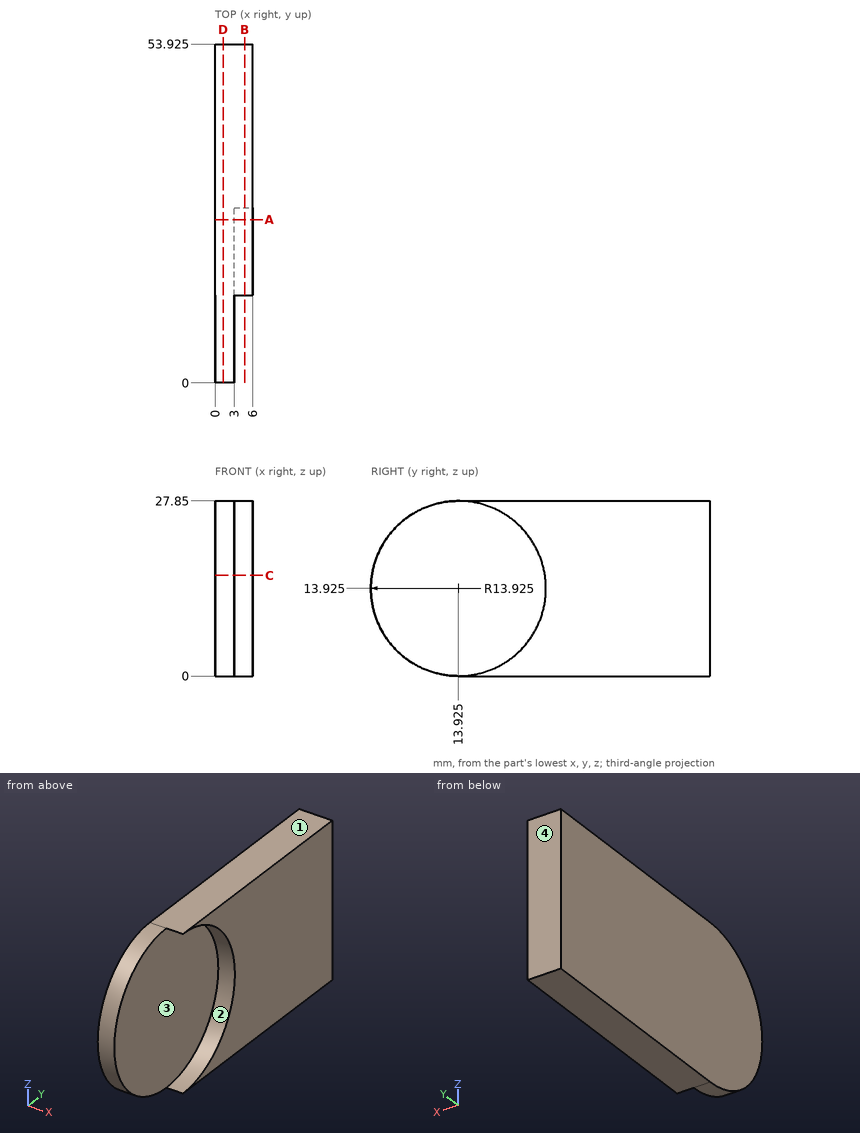
Can you work these out from the drawing? Everything is in mm from the part's minimum corner. Round coordinates to 2 decimals unless told otherwise and drop trailing zeros. Loops run counter-clockwise (first coordinate to the right, second up) from the corner with the lowest first, then second, coordinate; pieces in that order, holes last. Notation, with made-up numbers: M 65.25,53 L 89.25,53 A15 ccw 89.25,70 Z; hole C 59,73.25 d1. An arc over 180 degrees is marked long. Answer in a Markdown table with one row per item.
1. If we section it at A-A, the plane y = 26: Please give me the cut outline in (x, z), plus the area to 3 significant figures.
Established:
| item | result |
|---|---|
| outline | M 0,0 L 6,0 L 6,6.99 L 3,6.99 L 3,20.86 L 6,20.86 L 6,27.85 L 0,27.85 Z |
| area | 125 mm² |
2. Thinking about a two-plate mould opening in Z: for the marked faces 1, 2, 3 and 4, which applies, pulls with the +Z half, pulls with the -Z half, needs draft (parallel to the pull), parting line crosses it, or undercut?
Established:
| item | result |
|---|---|
| face 1 | pulls with the +Z half |
| face 2 | undercut |
| face 3 | undercut |
| face 4 | needs draft |
3. Please list where these lines run through material, in increasing order: line 1 (X direction, y = 10, z = 3.75); line 2 (Y direction, x = 4.5, z = 14.5) (3 decimals); line 3 (Y direction, x = 0.45, z = 26.25) (3 decimals). Write a range as from..to.
Established:
| item | result |
|---|---|
| line 1 | 0..3 |
| line 2 | 27.838..53.925 |
| line 3 | 7.444..53.925 |
4. If we section it at C-C, the plane z = 16: Please give me the cut outline in (x, y) (3 decimals), plus the area to 3 significant figures.
Established:
| item | result |
|---|---|
| outline | M 0,0.155 L 3,0.155 L 3,27.695 L 6,27.695 L 6,53.925 L 0,53.925 Z |
| area | 240 mm² |
5. I'm going to push flat-ended pins straight in: pin 1 Ø14 at (y, z) = (10, 7.5) entering from +X; pin 2 Ø1.5 at (x, z) = (1, 21) entering from -Y. Where does each tip first touch, or does it pass through?
Established:
| item | result |
|---|---|
| pin 1 | x = 3 |
| pin 2 | y = 1.52 |
6. If we section it at B-B, the plane x = 4.7: Please give me the cut outline in (y, z) (3 decimals), plus the area to 3 significant figures.
Established:
| item | result |
|---|---|
| outline | M 13.925,0 L 53.925,0 L 53.925,27.85 L 13.925,27.85 A13.925 cw Z |
| area | 809 mm² |
7. If we section it at D-D, the plane x = 1.25: Please give me the cut outline in (y, z) (3 decimals).
Established:
| item | result |
|---|---|
| outline | M 13.925,0 L 53.925,0 L 53.925,27.85 L 13.925,27.85 A13.925 ccw Z |
